Build history of the part. All positions in model axes, mm. A direction names the side the tool comes from. Round coordinates to 2 decimals unless told otherwise and drop trailing zeros. Write each loop counter-clockwise with the first axis right and the second up, starting at its lowest first coordinate (ties: lowest second). Pieces come first, ordered by that corner, then holes. Notation, with made-up numbers: M 82.5,83 L 102.5,83 A22 ccw 102.5,103 Z; hole C 24,1.5 d11. An arc over 180 degrees is marked long. Write item = value, one per line.
from build123d import *

# Parameters (mm, degrees)
F0_W     = 90
F0_H     = 90
F1_DEPTH = 45
F2_T     = -5
F3_D     = 70
F3_DEPTH = 10
F3_TIP   = 21.030121666
F6_D     = 20
F6_DEPTH = 12
F6_TIP   = 6.0086061903


with BuildPart() as f1:
    # F0 (on Front) → F1 (new body)
    with BuildSketch(Plane.XZ):
        Rectangle(F0_W, F0_H)
    extrude(amount=F1_DEPTH)

    # F2
    f2_openings = [f1.faces().sort_by_distance(p)[0] for p in [
        (45, -22.5, 0),
    ]]
    offset(amount=F2_T, openings=f2_openings)

    # F3
    with Locations(Plane(origin=(0, 0, 0), x_dir=(1, 0, 0), z_dir=(0, 1, 0))):
        with Locations((0, 0)):
            Hole(F3_D / 2, depth=F3_DEPTH)
            with Locations((0, 0, -(F3_DEPTH + F3_TIP / 2))):  # 118° drill point
                Cone(0, F3_D / 2, F3_TIP, mode=Mode.SUBTRACT)

    # F6
    with Locations(Plane(origin=(-45, 0, 0), x_dir=(0, -1, 0), z_dir=(-1, 0, 0))):
        with Locations((15.1247903705, 22.6402059197)):
            Hole(F6_D / 2, depth=F6_DEPTH)
            with Locations((0, 0, -(F6_DEPTH + F6_TIP / 2))):  # 118° drill point
                Cone(0, F6_D / 2, F6_TIP, mode=Mode.SUBTRACT)


solid = f1.part
1. Mould opens along Z. For faces 1 (the face through (-1, -45, 1)), 2 (the face through (-42.465, -16.427, 32.555)), 3 (the face through (-1, -22, -45)) say: pulls with the +Z half, pulls with the -Z half, needs draft (parallel to the pull), parting line crosses it, or undercut.
Responses:
face_1 = needs draft
face_2 = undercut
face_3 = pulls with the -Z half
2. Band-saw the part on B-B (z = -7). List the corners of the cut face in (x, y), plus the area to 3 significant figures.
Responses:
outline = M -45,-45 L 45,-45 L 45,-40 L -40,-40 L -40,-5 L -34.29,-5 L -34.29,0 L -45,0 Z; M 34.29,-5 L 45,-5 L 45,0 L 34.29,0 Z
area = 732 mm²
3. Band-saw the part on C-C (y = -15). List the corners of the cut face in (x, z), plus the area to 3 significant figures.
Responses:
outline = M -45,-45 L 45,-45 L 45,-40 L -40,-40 L -40,12.64 L -45,12.64 Z; M -45,32.64 L -40,32.64 L -40,40 L 45,40 L 45,45 L -45,45 Z
area = 1,200 mm²
4. Tool access for faces 4 (the face through (2, -22, -40)), 5 (the face through (-31, 0, 21)), 6 (the face through (28, -3, 21)): list every direction of +Z, -Z, +X, -X, +Y, -Y with a clear straight run to the whole face (end or side of a thin tool).
Responses:
face_4 = +X
face_5 = +Z, -Z, +X, -X, +Y
face_6 = +Y
5. Band-saw the part on A-A (x = 37). List the corners of the cut face in (y, z).
Responses:
outline = M -45,-45 L 0,-45 L 0,45 L -45,45 Z; hole M -40,-40 L -5,-40 L -5,40 L -40,40 Z
6. Band-saw the part on D-D (y = -28.5). List the corners of the cut face in (x, z), plus the area to 3 significant figures.
Responses:
outline = M -45,-45 L 45,-45 L 45,-40 L -40,-40 L -40,40 L 45,40 L 45,45 L -45,45 Z
area = 1,300 mm²
7. Probe probe 1 along Y at (x, z) = (-26, 26); probe 2 along Z at (x, y) = (10, -12); probe 3 along Z at (x, y) = (0, -3.6). List the from-to ranges inside material, lowest first.
Responses:
probe_1 = -45 to -40, -5 to 0
probe_2 = -45 to -40, 40 to 45
probe_3 = -45 to -35, 35 to 45
8. Flat gauge pins, fed straight in: pin 1 (10 mm diameter, centred on x = -5, z = -12, fed in from +Y); pin 2 (1 mm diameter, centred on x = -34, z = 11, fed in from +Y); pin 3 (10.5 mm diameter, centred on y = -25.5, z = 6, fed in from +X). Where does each tip first touch, or does it go through?
Responses:
pin_1 = -40
pin_2 = 0
pin_3 = -40
